Design review of the part built by this model. Coordinates are the model's own, in mm. Coordinates: 2 decimals unless noted, no trailing zeros. Loops run counter-clockwise (first coordinate to the right, second up) from the corner with the lowest first, then second, coordinate; pieces in that order, holes last. Notation, with made-up numbers: (-30, -38.75) - (6, -38.75) arc R13 cw to (6, -16.75) - close; hole circle Ø2 at (13.5, -8). An arc over 180 degrees is marked (long way). Use one line per item in the form item = value. Start each with the question number.
(1) Add section B-B (z = 64.5). State the section outline as (x, y) points (3 decimals), plus the area to 3 significant figures.
(2) Add section A-A (z = 37). State the section outline as (x, y) points (3 decimals), plus the area to 3 significant figures.
(3) The part is to be moulded in two halves that separate along X. For faces 1 (the face through (-2.9, -13.06, 17.26)), 2 (the face through (14.91, 4.69, 52.25)), 3 (the face through (-7, -12, 0)), say which applies: pulls with the +X half, pulls with the -X half, needs draft (parallel to the pull), parting line crosses it, or undercut.
(4) For L1, parallel to Y at x = 4, z = 14; L2, parallel to X at y = -12, z = 63; L3, parallel to Y at x = 10.5, z = 45 (3 decimals), list the stretches that pass through material, from the lowest coordinate up.
(5) Clearance check with flat-ended pins moving along their axes: pin 1 Ø10 at (y, z) = (7, 34) entering from -X; pin 2 Ø1 at (y, z) = (6, 31) entering from -X; pin 3 Ø4 at (y, z) = (-6.5, 33) entering from +X. State where each tip first meets the part, or that it passes through.
```python
from build123d import *

# Parameters (mm, degrees)
F2_R    = 1
F3_SIZE = 1


with BuildPart() as f1:
    # F0 (on Front) → F1 (revolve)
    with BuildSketch(Plane.XZ):
        Polygon((15.875, 0), (15.875, 35), (15.375, 70), (13.125, 70), (13.125, 35), (13.625, 0), align=None)
    revolve(axis=Axis((0, 0, 29.460958), (0, 0, 1)))

    # F2
    f2_edges = [f1.edges().sort_by_distance(p)[0] for p in [
        (-15.375, 0, 70),
        (-13.125, 0, 70),
    ]]
    fillet(f2_edges, radius=F2_R)

    # F3
    f3_edges = [f1.edges().sort_by_distance(p)[0] for p in [
        (-15.875, 0, 0),
    ]]
    chamfer(f3_edges, length=F3_SIZE)


solid = f1.part
```
Computed values:
q1.outline = circle Ø30.907 at (0, 0); hole circle Ø26.25 at (0, 0)
q1.area = 209 mm^2
q2.outline = circle Ø31.693 at (0, 0); hole circle Ø26.25 at (0, 0)
q2.area = 248 mm^2
q3.face_1 = undercut
q3.face_2 = parting line crosses it
q3.face_3 = needs draft
q4.L1 = -15.36 to -12.82, 12.82 to 15.36
q4.L2 = -9.77 to -5.32, 5.32 to 9.77
q4.L3 = -11.715 to -7.875, 7.875 to 11.715
q5.pin_1 = -15.75
q5.pin_2 = -14.89
q5.pin_3 = 15.22
